Here's how the part is built. I have some questions about the finished solid (model axes, mm). Face numbers are marked on the shaded views. A direction names the side the tool comes from. Round coordinates to 2 decimals unless told otherwise and drop trailing zeros. Write each loop counter-clockwise with the first axis right and the second up, starting at its lowest first coordinate (ties: lowest second). Pieces come first, ordered by that corner, then holes. Notation, with made-up numbers: (64, 80.25) -> (85, 80.25) arc R22 ccw to (85, 118.25) -> close; hole circle Ø1 at (-25.5, -25.5). An arc over 180 degrees is marked (long way). Answer as CSV lines item,"result".
```python
from build123d import *

# Parameters (mm, degrees)
F0_W     = 120
F0_H     = 120
F1_DEPTH = 3
F2_W     = 52
F2_H     = 52
F3_DEPTH = 25
F2_W_2   = 120
F2_H_2   = 120
F2_W_3   = 70
F2_H_3   = 70
F2_R     = 2.5
F4_DEPTH = 37
F5_W     = 120
F5_H     = 120
F5_W_2   = 114
F5_H_2   = 114
F5_W_3   = 52
F5_H_3   = 52
F6_DEPTH = 3


with BuildPart() as f1:
    # F0 (on Top) → F1 (new body)
    with BuildSketch(Plane.XY):
        Rectangle(F0_W, F0_H)
    extrude(amount=F1_DEPTH)

    # F2 (on face) → F3 (cut)
    with BuildSketch(Plane.XY.offset(3)):
        Rectangle(F2_W, F2_H)
    extrude(amount=-F3_DEPTH, mode=Mode.SUBTRACT)

    # F2 (on face) → F4 (join)
    with BuildSketch(Plane.XY.offset(3)):
        Rectangle(F2_W_2, F2_H_2)
        Polygon((-57, -57), (-57, -35), (-57, 35), (-57, 57), (-35, 57), (35, 57), (57, 57), (57, 35), (57, -35), (57, -57), (35, -57), (-35, -57), align=None, mode=Mode.SUBTRACT)
        Rectangle(F2_W_3, F2_H_3)
        Rectangle(F2_W, F2_H, mode=Mode.SUBTRACT)
        with Locations((46, 46)):
            Circle(F2_R)
        with Locations((0, 46)):
            Circle(F2_R)
        with Locations((-46, 46)):
            Circle(F2_R)
        with Locations((-46, 0)):
            Circle(F2_R)
        with Locations((-46, -46)):
            Circle(F2_R)
        with Locations((0, -46)):
            Circle(F2_R)
        with Locations((46, -46)):
            Circle(F2_R)
        with Locations((46, 0)):
            Circle(F2_R)
    extrude(amount=F4_DEPTH)

    # F5 (on face) → F6 (join)
    with BuildSketch(Plane.XY.offset(40)):
        Rectangle(F5_W, F5_H)
        Rectangle(F5_W_2, F5_H_2, mode=Mode.SUBTRACT)
        Rectangle(F5_W_2, F5_H_2)
        Rectangle(F5_W_3, F5_H_3, mode=Mode.SUBTRACT)
    extrude(amount=F6_DEPTH)


solid = f1.part
```
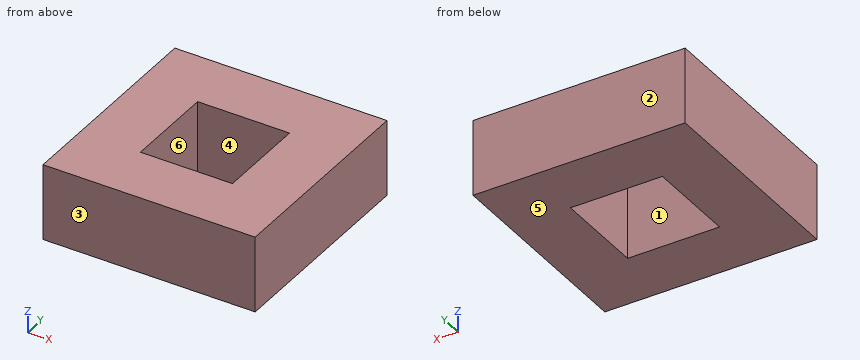
1. If we mould it in two halves opening along Y, with no side actions, what happens to the marked faces 3, 4, 5 and 6? For each: released by +Y, released by -Y, zero draft, split by the parting line, or undercut.
Numbers:
face 3,"released by -Y"
face 4,"undercut"
face 5,"zero draft"
face 6,"undercut"
2. If I drill on line 1 (X direction, y = -17, z = 17.5); line 2 (Y direction, x = 27, z = 18), over which ranges is the centre line in solid material (lowest first)?
Numbers:
line 1,"x = -60 to -57, -35 to -26, 26 to 35, 57 to 60"
line 2,"y = -60 to -57, -35 to 35, 57 to 60"
3. Suppose I cut it at A-A on x = 14. Please give me the cut outline in (y, z), and give its area (3 significant figures).
Numbers:
outline,"(-60, 0) -> (-26, 0) -> (-26, 43) -> (-60, 43) -> close; (26, 0) -> (60, 0) -> (60, 43) -> (26, 43) -> close; hole (-57, 3) -> (-35, 3) -> (-35, 40) -> (-57, 40) -> close; hole (35, 3) -> (57, 3) -> (57, 40) -> (35, 40) -> close"
area,"1,300 mm^2"
4. Suppose I cut it at D-D on x = 29. Please give me the cut outline in (y, z), and give its area (3 significant figures).
Numbers:
outline,"(-60, 0) -> (60, 0) -> (60, 43) -> (-60, 43) -> close; hole (-57, 3) -> (-35, 3) -> (-35, 40) -> (-57, 40) -> close; hole (35, 3) -> (57, 3) -> (57, 40) -> (35, 40) -> close"
area,"3,530 mm^2"
5. On a 3-axis mill with a long thin cutter (end or side, diameter ignored), from which of +Z, -Z, +X, -X, +Y, -Y can I reach the whole of each face in a straight line? I mean the marked faces 1 and 2. Say none if no direction works.
Numbers:
face 1,"+Z, -Z"
face 2,"+Z, -Z, +X, -X, +Y"
6. Suppose I cut it at C-C on y = 0. Please give me the cut outline in (x, z).
Numbers:
outline,"(-60, 0) -> (-26, 0) -> (-26, 43) -> (-60, 43) -> close; (26, 0) -> (60, 0) -> (60, 43) -> (26, 43) -> close; hole (-57, 3) -> (-48.5, 3) -> (-48.5, 40) -> (-57, 40) -> close; hole (-43.5, 3) -> (-35, 3) -> (-35, 40) -> (-43.5, 40) -> close; hole (35, 3) -> (43.5, 3) -> (43.5, 40) -> (35, 40) -> close; hole (48.5, 3) -> (57, 3) -> (57, 40) -> (48.5, 40) -> close"
7. Suppose I cut it at B-B on z = 32.5. Count the separate pieces of the cut face and the enclosed holes in it, and give its area (3 significant figures).
Numbers:
separate pieces,"10"
enclosed holes,"2"
area,"3,760 mm^2"
